Could you check a few things on this model? Use its own coordinates, in mm. A direction names the side the tool comes from. Round coordinates to 2 decimals unless told otherwise and drop trailing zeros. Loops run counter-clockwise (first coordinate to the right, second up) from the corner with the lowest first, then second, coordinate; pieces in that order, holes last.
from build123d import *

# Parameters (mm, degrees)
SKETCH_1_W      = 28
SKETCH_1_H      = 20
SKETCH_1_R      = 1
SKETCH_1_R_2    = 8
EXTRUDE_1_DEPTH = 4
SKETCH_2_W      = 3
SKETCH_2_H      = 20
EXTRUDE_2_DEPTH = 10
SKETCH_3_R      = 4
SKETCH_3_R_2    = 3
EXTRUDE_3_DEPTH = 1
SKETCH_4_R      = 3
EXTRUDE_4_DEPTH = 6
CHAMFER_1_SIZE  = 4


with BuildPart() as part:
    # 草图1 → 凸台-拉伸1 (new body)
    with BuildSketch(Plane.XY):
        Rectangle(SKETCH_1_W, SKETCH_1_H)
        with Locations((7.7, -7.7)):
            Circle(SKETCH_1_R, mode=Mode.SUBTRACT)
        Circle(SKETCH_1_R_2, mode=Mode.SUBTRACT)
        with Locations((-7.7, -7.7)):
            Circle(SKETCH_1_R, mode=Mode.SUBTRACT)
        with Locations((-7.7, 7.7)):
            Circle(SKETCH_1_R, mode=Mode.SUBTRACT)
        with Locations((7.7, 7.7)):
            Circle(SKETCH_1_R, mode=Mode.SUBTRACT)
    extrude(amount=EXTRUDE_1_DEPTH)

    # 草图2 → 凸台-拉伸2 (add)
    with BuildSketch(Plane.XY.offset(4)):
        with Locations((-12.5, 0)):
            Rectangle(SKETCH_2_W, SKETCH_2_H)
        with Locations((12.5, 0)):
            Rectangle(SKETCH_2_W, SKETCH_2_H)
    extrude(amount=EXTRUDE_2_DEPTH)

    # 草图3 → 凸台-拉伸3 (add)
    # profile 1 of 2: a face of its own
    with BuildSketch(Plane(origin=(14, 0, 0), x_dir=(0, 0, -1), z_dir=(1, 0, 0))):
        with Locations(Location((-7, 0, 0), (0, 0, 90))):
            Circle(SKETCH_3_R)
        with Locations((-7, 0)):
            Circle(SKETCH_3_R_2, mode=Mode.SUBTRACT)
    # profile 2 of 2: a face of its own
    with BuildSketch(Plane(origin=(14, 0, 0), x_dir=(0, 0, -1), z_dir=(1, 0, 0))):
        with Locations((-7, 0)):
            Circle(SKETCH_3_R_2)
    extrude_3 = extrude(amount=EXTRUDE_3_DEPTH)

    # 草图4 → 凸台-拉伸4 (add)
    with BuildSketch(Plane(origin=(15, 0, 0), x_dir=(0, 0, -1), z_dir=(1, 0, 0))):
        with Locations(Location((-7, 0, 0), (0, 0, 90))):
            Circle(SKETCH_4_R)
    extrude_4 = extrude(amount=EXTRUDE_4_DEPTH)

    # 倒角1
    chamfer_1_edges = [part.edges().sort_by_distance(p)[0] for p in [
        (-12.5, -10, 14),
        (-12.5, 10, 14),
        (12.5, 10, 14),
        (12.5, -10, 14),
    ]]
    chamfer(chamfer_1_edges, length=CHAMFER_1_SIZE)

    # 镜向2: 凸台-拉伸3, 凸台-拉伸4 across plane
    add(extrude_3.mirror(Plane(origin=(0, 0, 0), x_dir=(0, 0, 1), z_dir=(1, 0, 0))))
    add(extrude_4.mirror(Plane(origin=(0, 0, 0), x_dir=(0, 0, 1), z_dir=(1, 0, 0))))


solid = part.part
Item 1: We'd pull the mould along X, two halves only. Please class faces 6 (the flat face through (12, 8, 12)), 7 (the cylindrical face through (-6.776, -8.083, 1.972)), 8 (the flat face through (-15, 1, 10)), 9 (the cylindrical face through (-6.776, 7.317, 1.972)): released by +X, released by -X, zero draft, split by the parting line, or undercut.
Results list:
face 6: zero draft
face 7: undercut
face 8: released by -X
face 9: undercut
Item 2: If I drill on line 1 along X through (y, z) = (9, 5.75); line 2 along X through (y, z) = (2.75, 9); line 3 along X through (y, z) = (-7, 2.75), over which ranges is the centre line in solid material (lowest first)?
Results list:
line 1: x = -14 to -11, 11 to 14
line 2: x = -15 to -11, 11 to 15
line 3: x = -14 to -8.41, -6.99 to -3.87, 3.87 to 6.99, 8.41 to 14
Item 3: If we section it at D-D, the plane z = 11.5: Please give me the cut outline in (x, y), then the cut area to 3 significant figures.
Results list:
outline: (-14, -8.5) - (-11, -8.5) - (-11, 8.5) - (-14, 8.5) - close; (11, -8.5) - (14, -8.5) - (14, 8.5) - (11, 8.5) - close
area: 102 mm2
Item 4: Will these pins go through, and if not, where does the flat tip stop? pin 1 (2.5 mm diameter, centred on x = -7.7, y = -7.7, fed in from +Z); pin 2 (1 mm diameter, centred on y = -5.5, z = 5.5, fed in from -X).
Results list:
pin 1: stops at z = 4
pin 2: stops at x = -14
Item 5: If we section it at C-C, the plane y = 2.25: Please give me the cut outline in (x, z), then the cut area to 3 significant figures.
Results list:
outline: (-21, 5.02) - (-15, 5.02) - (-15, 3.69) - (-14, 3.69) - (-14, 0) - (-7.68, 0) - (-7.68, 4) - (-11, 4) - (-11, 14) - (-14, 14) - (-14, 10.31) - (-15, 10.31) - (-15, 8.98) - (-21, 8.98) - close; (7.68, 0) - (14, 0) - (14, 3.69) - (15, 3.69) - (15, 5.02) - (21, 5.02) - (21, 8.98) - (15, 8.98) - (15, 10.31) - (14, 10.31) - (14, 14) - (11, 14) - (11, 4) - (7.68, 4) - close
area: 171 mm2
Item 6: If we section it at B-B, the plane x = -2: Please give me the cut outline in (y, z), then the cut area to 3 significant figures.
Results list:
outline: (-10, 0) - (-7.75, 0) - (-7.75, 4) - (-10, 4) - close; (7.75, 0) - (10, 0) - (10, 4) - (7.75, 4) - close
area: 18.0 mm2
Item 7: For faces 1 (the cylindrical face through (14.493, -3.996, 7.176)), 2 (the flat face through (0, 10, 3)), 3 (the flat face through (11, 0, 9)), 4 (the cylindrical face through (-14.493, -3.996, 7.176)), 5 (the flat face through (0, -9, 0)), which set-ups out of +Z, -Z, +X, -X, +Y, -Y let a thin tool reach every point of the face, with its end or its side?
Results list:
face 1: +X
face 2: +Z, -Z, +X, -X, +Y
face 3: +Z, +Y, -Y
face 4: -X
face 5: -Z, +X, -X, +Y, -Y
Item 8: If we section it at A-A, the plane z = 7: Please give me the cut outline in (x, y), then the cut area to 3 significant figures.
Results list:
outline: (-21, -3) - (-15, -3) - (-15, -4) - (-14, -4) - (-14, -10) - (-11, -10) - (-11, 10) - (-14, 10) - (-14, 4) - (-15, 4) - (-15, 3) - (-21, 3) - close; (11, -10) - (14, -10) - (14, -4) - (15, -4) - (15, -3) - (21, -3) - (21, 3) - (15, 3) - (15, 4) - (14, 4) - (14, 10) - (11, 10) - close
area: 208 mm2
